```python
from build123d import *

# Parameters (mm, degrees)
SKICA1_W                 = 30
SKICA1_H                 = 150
P_IDAT_VYSUNUT_M1_DEPTH  = 5
ZAOBLIT1_R               = 10
SKICA2_W                 = 13
SKICA2_H                 = 25
ODEBRAT_VYSUNUT_M1_DEPTH = 154.05227865
SKICA3_R                 = 0.5
ODEBRAT_VYSUNUT_M2_DEPTH = 154.05227865
ODEBRAT_VYSUNUT_M3_DEPTH = 2
SKICA5_R                 = 0.5
ODEBRAT_VYSUNUT_M4_DEPTH = 154
SKICA6_R                 = 3.75
ODEBRAT_VYSUNUT_M5_DEPTH = 2
SKICA7_W                 = 7.5
SKICA7_H                 = 8
ODEBRAT_VYSUNUT_M6_DEPTH = 154.05227865


with BuildPart() as part:
    # Skica1 → Přidat vysunutím1 (new body)
    with BuildSketch(Plane.XY):
        with Locations((15, 75)):
            Rectangle(SKICA1_W, SKICA1_H)
    extrude(amount=P_IDAT_VYSUNUT_M1_DEPTH)

    # Zaoblit1
    zaoblit1_edges = [part.edges().sort_by_distance(p)[0] for p in [
        (0, 150, 2.5),
        (30, 150, 2.5),
        (30, 0, 2.5),
        (0, 0, 2.5),
    ]]
    fillet(zaoblit1_edges, radius=ZAOBLIT1_R)

    # Skica2 → Odebrat vysunutím1 (cut, through all)
    with BuildSketch(Plane.XY.offset(5)):
        with Locations((15, 127.5)):
            Rectangle(SKICA2_W, SKICA2_H)
    extrude(amount=-ODEBRAT_VYSUNUT_M1_DEPTH, mode=Mode.SUBTRACT)

    # Skica3 → Odebrat vysunutím2 (cut, through all)
    with BuildSketch(Plane.XY.offset(5)):
        with Locations((15, 141.5)):
            Circle(SKICA3_R)
        with Locations(Location((15, 113.5, 0), (0, 0, 180))):
            Circle(SKICA3_R)
    extrude(amount=-ODEBRAT_VYSUNUT_M2_DEPTH, mode=Mode.SUBTRACT)

    # Skica4 → Odebrat vysunutím3 (cut)
    with BuildSketch(Plane.XY.offset(5)):
        Polygon((18.40625, 20), (11.59375, 20), (13, 5), (17, 5), align=None)
        Polygon((18.5, 21), (11.5, 21), (11.59375, 20), (18.40625, 20), align=None)
        Polygon((11.59375, 20), (11.5, 21), (11.772727273, 24), (8, 24), (8, 20), align=None)
        Polygon((11.772727273, 24), (11.5, 21), (18.5, 21), (18.227272727, 24), align=None)
        Polygon((18.227272727, 24), (18.5, 21), (18.40625, 20), (22, 20), (22, 24), align=None)
        with BuildLine():
            ThreePointArc((22, 24), (24, 22), (22, 20))
            Line((22, 20), (22, 24))
        make_face()
        with BuildLine():
            Line((8, 24), (8, 20))
            ThreePointArc((8, 20), (6, 22), (8, 24))
        make_face()
        Polygon((13.5, 43), (11.772727273, 24), (18.227272727, 24), (16.5, 43), align=None)
    extrude(amount=-ODEBRAT_VYSUNUT_M3_DEPTH, mode=Mode.SUBTRACT)

    # Skica5 → Odebrat vysunutím4 (cut, through all)
    with BuildSketch(Plane.XY.offset(3)):
        with Locations((15, 36.2)):
            Circle(SKICA5_R)
        with Locations((15, 9.7)):
            Circle(SKICA5_R)
    extrude(amount=-ODEBRAT_VYSUNUT_M4_DEPTH, mode=Mode.SUBTRACT)

    # Skica6 → Odebrat vysunutím5 (cut)
    with BuildSketch(Plane.XY.offset(3)):
        with Locations((15, 22)):
            Circle(SKICA6_R)
    extrude(amount=-ODEBRAT_VYSUNUT_M5_DEPTH, mode=Mode.SUBTRACT)

    # Skica7 → Odebrat vysunutím6 (cut, through all)
    with BuildSketch(Plane.XY.offset(5)):
        with Locations((7.84375, 16)):
            Rectangle(SKICA7_W, SKICA7_H)
    extrude(amount=-ODEBRAT_VYSUNUT_M6_DEPTH, mode=Mode.SUBTRACT)


solid = part.part
```
Input: part model. Units: mm. Frame: model coordinates. A direction names the side the tool comes from. Coordinates: 2 decimals unless noted, no trailing zeros. Loops run counter-clockwise (first coordinate to the right, second up) from the corner with the lowest first, then second, coordinate; pieces in that order, holes last. Notation, with made-up numbers: M 49,12 L 75,12 A21 cw 75,19 Z; hole C -29.75,47 d5. An arc over 180 degrees is marked long. One line per item, written item: value.
(1) Section A-A (y = 131.5). Output: boundary loops of the cut face in (x, z), and give its area (3 significant figures).
Filled in:
outline: M 0,0 L 8.5,0 L 8.5,5 L 0,5 Z; M 21.5,0 L 30,0 L 30,5 L 21.5,5 Z
area: 85.0 mm^2
(2) Pin query (flat end, axial travel): pin 1 (4 mm diameter, centred on x = 14, y = 22, fed in from +Z). Return the tip coordinate at first contact, or that it passes through.
Filled in:
pin 1: z = 1
(3) Line query: line 1 along Y through (x, z) = (14.25, 4.5); line 2 along Y through (x, z) = (11, 1); line 3 along X through (y, z) = (122, 3.8). Output: solid intervals per line, ascending. Write a range as from..to.
Filled in:
line 1: 0..5, 43..115, 140..150
line 2: 0..12, 20..115, 140..150
line 3: 0..8.5, 21.5..30
(4) Pull-direction query (Y, two-part tool) for faces 4 (the flat face through (15, 0, 2)), 5 (the flat face through (8, 12, 3)), 6 (the flat face through (15, 22, 1)), 7 (the flat face through (15, 76, 5)); classes: +Y half, -Y half, draft (parallel to the pull), parting line (faces both ways), or undercut.
Filled in:
face 4: -Y half
face 5: undercut
face 6: undercut
face 7: draft
(5) Reachability of faces 1 (the flat face through (8.5, 127, 3)), 2 (the cylindrical face through (27.15, 146.99, 2.54)), 3 (the cylindrical face through (14.19, 18.34, 2.01)) from +Z, -Z, +X, -X, +Y, -Y: full face, straight path, thin tool, end or side. Return the list, or none.
Filled in:
face 1: +Z, -Z
face 2: +Z, -Z, +X, +Y
face 3: +Z
